Can you work these out from the model? Positions are in its coordinate system, mm. A direction names the side the tool comes from. Coordinates: 2 decimals unless noted, no trailing zeros. Order: outer loops, then holes, each group sorted by start corner. A loop starts at its lowest first (then second) coordinate and runs counter-clockwise, first axis right, second up. Notation, with made-up numbers: (-20, 87) -> (-15, 87) arc R21 cw to (-15, 120) -> close; hole circle Ø10 at (-6.5, 23). An arc over 180 degrees is marked (long way). Answer as CSV lines item,"result".
from build123d import *

# Parameters (mm, degrees)
SKETCH1_W           = 300
SKETCH1_H           = 200
BOSS_EXTRUDE1_DEPTH = 6
SKETCH6_R           = 4
CUT_EXTRUDE2_DEPTH  = 361.605047108
FILLET1_R           = 6.35
SKETCH2_R           = 1.5
CUT_EXTRUDE1_DEPTH  = 361.605047108
SKETCH16_R          = 2.65
M5_THROUGH_DEPTH    = 358.420816406
SKETCH9_R           = 1.5
CUT_EXTRUDE3_DEPTH  = 361.605047108
SKETCH10_R          = 1.5
CUT_EXTRUDE5_DEPTH  = 361.605047108
SKETCH17_R          = 1.6
M3_THROUGH_DEPTH    = 268.189599912
FILLET2_R           = 6.35
MOVE_FACE1_BY       = 0.08
MOVE_FACE1_2_BY     = 0.08
MOVE_FACE1_3_BY     = 0.08
MOVE_FACE1_4_BY     = 0.08
MOVE_FACE1_5_BY     = 0.08
MOVE_FACE1_6_BY     = 0.08
MOVE_FACE1_7_BY     = 0.08
MOVE_FACE1_8_BY     = 0.08
MOVE_FACE1_9_BY     = 0.08
MOVE_FACE1_10_BY    = 0.08
MOVE_FACE1_11_BY    = 0.08
MOVE_FACE1_12_BY    = 0.08
MOVE_FACE1_13_BY    = 0.08
MOVE_FACE1_14_BY    = 0.08
MOVE_FACE1_15_BY    = 0.08
MOVE_FACE1_16_BY    = 0.08
MOVE_FACE1_17_BY    = 0.08
MOVE_FACE1_18_BY    = 0.08
MOVE_FACE1_19_BY    = 0.08
MOVE_FACE1_20_BY    = 0.08
MOVE_FACE1_21_BY    = 0.08
MOVE_FACE1_22_BY    = 0.08
MOVE_FACE1_23_BY    = 0.08
MOVE_FACE1_24_BY    = 0.08
MOVE_FACE1_25_BY    = 0.08
MOVE_FACE1_26_BY    = 0.08


with BuildPart() as part:
    # Sketch1 → Boss-Extrude1 (new body)
    with BuildSketch(Plane(origin=(0, 0, 0), x_dir=(1, 0, 0), z_dir=(0, 1, 0))):
        with Locations((150, 100)):
            Rectangle(SKETCH1_W, SKETCH1_H)
    extrude(amount=BOSS_EXTRUDE1_DEPTH)

    # Sketch6 → Cut-Extrude2 (cut, through all)
    with BuildSketch(Plane(origin=(0, 6, 0), x_dir=(1, 0, 0), z_dir=(0, 1, 0))):
        with Locations(Location((150, 118.651, 0), (0, 0, 270))):
            Circle(SKETCH6_R)
    extrude(amount=-CUT_EXTRUDE2_DEPTH, mode=Mode.SUBTRACT)

    # Fillet1
    fillet1_edges = [part.edges().sort_by_distance(p)[0] for p in [
        (0, 3, -200),
        (300, 3, -200),
        (300, 3, 0),
        (0, 3, 0),
    ]]
    fillet(fillet1_edges, radius=FILLET1_R)

    # Sketch2 → Cut-Extrude1 (cut, through all)
    with BuildSketch(Plane(origin=(0, 6, 0), x_dir=(1, 0, 0), z_dir=(0, 1, 0))):
        with Locations(Location((6.35, 174.6, 0), (0, 0, 270))):
            Circle(SKETCH2_R)
        with Locations(Location((6.35, 49.9999, 0), (0, 0, 270))):
            Circle(SKETCH2_R)
        with Locations(Location((249.2, 75.3999, 0), (0, 0, 270))):
            Circle(SKETCH2_R)
        with Locations(Location((50.8, 75.3999, 0), (0, 0, 270))):
            Circle(SKETCH2_R)
        with Locations(Location((293.65, 49.9999, 0), (0, 0, 270))):
            Circle(SKETCH2_R)
        with Locations(Location((50.8, 24.5999, 0), (0, 0, 270))):
            Circle(SKETCH2_R)
        with Locations(Location((249.2, 24.5999, 0), (0, 0, 270))):
            Circle(SKETCH2_R)
        with Locations(Location((25.4, 193.65, 0), (0, 0, 270))):
            Circle(SKETCH2_R)
        with Locations(Location((274.6, 193.65, 0), (0, 0, 270))):
            Circle(SKETCH2_R)
        with Locations(Location((293.65, 174.6, 0), (0, 0, 270))):
            Circle(SKETCH2_R)
    extrude(amount=-CUT_EXTRUDE1_DEPTH, mode=Mode.SUBTRACT)

    # Sketch16 → M5_through (cut, through all)
    with BuildSketch(Plane(origin=(0, 6, -5.8), x_dir=(1, 0, 0), z_dir=(0, -1, 0))):
        with Locations(Location((118.25, -18.651, 0), (0, 0, 270))):
            Circle(SKETCH16_R)
        with Locations(Location((118.25, -0.55096, 0), (0, 0, 270))):
            Circle(SKETCH16_R)
        with Locations(Location((139.416666667, -0.55096, 0), (0, 0, 270))):
            Circle(SKETCH16_R)
        with Locations(Location((160.583333333, -0.55096, 0), (0, 0, 270))):
            Circle(SKETCH16_R)
        with Locations(Location((181.75, -0.55096, 0), (0, 0, 270))):
            Circle(SKETCH16_R)
        with Locations(Location((181.75, -18.651, 0), (0, 0, 270))):
            Circle(SKETCH16_R)
    extrude(amount=M5_THROUGH_DEPTH, mode=Mode.SUBTRACT)

    # Sketch9 → Cut-Extrude3 (cut, through all)
    with BuildSketch(Plane(origin=(0, 6, 0), x_dir=(-1, 0, 0), z_dir=(0, 1, 0))):
        with Locations(Location((-118.25, -15.40098, 0), (0, 0, 90))):
            Circle(SKETCH9_R)
        with Locations(Location((-150, -6.35096, 0), (0, 0, 90))):
            Circle(SKETCH9_R)
        with Locations(Location((-181.75, -15.40098, 0), (0, 0, 90))):
            Circle(SKETCH9_R)
    extrude(amount=-CUT_EXTRUDE3_DEPTH, mode=Mode.SUBTRACT)

    # Sketch10 → Cut-Extrude5 (cut, through all)
    with BuildSketch(Plane(origin=(0, 6, 0), x_dir=(1, 0, 0), z_dir=(0, 1, 0))):
        with Locations(Location((150, 156.751, 0), (0, 0, 270))):
            Circle(SKETCH10_R)
        with Locations(Location((182.995567884, 137.701, 0), (0, 0, 270))):
            Circle(SKETCH10_R)
        with Locations(Location((182.995567884, 99.601, 0), (0, 0, 270))):
            Circle(SKETCH10_R)
        with Locations(Location((150, 80.551, 0), (0, 0, 270))):
            Circle(SKETCH10_R)
        with Locations(Location((117.004432116, 99.601, 0), (0, 0, 270))):
            Circle(SKETCH10_R)
        with Locations(Location((117.004432116, 137.701, 0), (0, 0, 270))):
            Circle(SKETCH10_R)
        with Locations(Location((105.55, 30.801, 0), (0, 0, 270))):
            Circle(SKETCH10_R)
        with Locations(Location((105.55, 6.35, 0), (0, 0, 270))):
            Circle(SKETCH10_R)
        with Locations(Location((194.45, 6.35, 0), (0, 0, 90))):
            Circle(SKETCH10_R)
        with Locations(Location((194.45, 30.801, 0), (0, 0, 90))):
            Circle(SKETCH10_R)
        with BuildLine():
            Line((124.6, 75.583146559), (124.6, 37.151))
            Line((124.6, 37.151), (92.85, 37.151))
            Line((92.85, 37.151), (92.85, 0))
            Line((92.85, 0), (0, 0))
            Line((0, 0), (0, 200))
            Line((0, 200), (300, 200))
            Line((300, 200), (300, 0))
            Line((300, 0), (207.15, 0))
            Line((207.15, 0), (207.15, 37.151))
            Line((207.15, 37.151), (175.4, 37.151))
            Line((175.4, 37.151), (175.4, 75.583146559))
            ThreePointArc((175.4, 75.583146559), (150, 168.651), (124.6, 75.583146559))
        make_face()
    extrude(amount=-CUT_EXTRUDE5_DEPTH, mode=Mode.SUBTRACT)

    # Sketch17 → M3-through (cut, through all)
    with BuildSketch(Plane(origin=(0, 6, 0), x_dir=(1, 0, 0), z_dir=(0, 1, 0))):
        with Locations(Location((188.1, 118.651, 0), (0, 0, 270))):
            Circle(SKETCH17_R)
        with Locations(Location((169.05, 85.655432116, 0), (0, 0, 270))):
            Circle(SKETCH17_R)
        with Locations(Location((130.95, 85.655432116, 0), (0, 0, 270))):
            Circle(SKETCH17_R)
        with Locations(Location((111.9, 118.651, 0), (0, 0, 270))):
            Circle(SKETCH17_R)
        with Locations(Location((130.95, 151.646567884, 0), (0, 0, 270))):
            Circle(SKETCH17_R)
        with Locations(Location((169.05, 151.646567884, 0), (0, 0, 270))):
            Circle(SKETCH17_R)
    extrude(amount=-M3_THROUGH_DEPTH, mode=Mode.SUBTRACT)

    # Fillet2
    fillet2_edges = [part.edges().sort_by_distance(p)[0] for p in [
        (175.4, 3, -75.583146559),
        (124.6, 3, -75.583146559),
        (124.6, 3, -37.151),
        (92.85, 3, -37.151),
        (92.85, 3, 0),
        (207.15, 3, 0),
        (207.15, 3, -37.151),
        (175.4, 3, -37.151),
    ]]
    fillet(fillet2_edges, radius=FILLET2_R)

    # Move Face1: a curved face moved outward by 0.08
    add(Solid.thicken(part.faces().sort_by_distance((150, 3, -122.651))[0], MOVE_FACE1_BY))

    # Move Face1 2: a curved face moved outward by 0.08
    add(Solid.thicken(part.faces().sort_by_distance((118.25, 3, -21.801))[0], MOVE_FACE1_2_BY))

    # Move Face1 3: a curved face moved outward by 0.08
    add(Solid.thicken(part.faces().sort_by_distance((118.25, 3, -3.70096))[0], MOVE_FACE1_3_BY))

    # Move Face1 4: a curved face moved outward by 0.08
    add(Solid.thicken(part.faces().sort_by_distance((139.416666667, 3, -3.70096))[0], MOVE_FACE1_4_BY))

    # Move Face1 5: a curved face moved outward by 0.08
    add(Solid.thicken(part.faces().sort_by_distance((160.583333333, 3, -3.70096))[0], MOVE_FACE1_5_BY))

    # Move Face1 6: a curved face moved outward by 0.08
    add(Solid.thicken(part.faces().sort_by_distance((181.75, 3, -3.70096))[0], MOVE_FACE1_6_BY))

    # Move Face1 7: a curved face moved outward by 0.08
    add(Solid.thicken(part.faces().sort_by_distance((181.75, 3, -21.801))[0], MOVE_FACE1_7_BY))

    # Move Face1 8: a curved face moved outward by 0.08
    add(Solid.thicken(part.faces().sort_by_distance((118.25, 3, -16.90098))[0], MOVE_FACE1_8_BY))

    # Move Face1 9: a curved face moved outward by 0.08
    add(Solid.thicken(part.faces().sort_by_distance((150, 3, -7.85096))[0], MOVE_FACE1_9_BY))

    # Move Face1 10: a curved face moved outward by 0.08
    add(Solid.thicken(part.faces().sort_by_distance((181.75, 3, -16.90098))[0], MOVE_FACE1_10_BY))

    # Move Face1 11: a curved face moved outward by 0.08
    add(Solid.thicken(part.faces().sort_by_distance((150, 3, -158.251))[0], MOVE_FACE1_11_BY))

    # Move Face1 12: a curved face moved outward by 0.08
    add(Solid.thicken(part.faces().sort_by_distance((182.995567884, 3, -139.201))[0], MOVE_FACE1_12_BY))

    # Move Face1 13: a curved face moved outward by 0.08
    add(Solid.thicken(part.faces().sort_by_distance((182.995567884, 3, -101.101))[0], MOVE_FACE1_13_BY))

    # Move Face1 14: a curved face moved outward by 0.08
    add(Solid.thicken(part.faces().sort_by_distance((150, 3, -82.051))[0], MOVE_FACE1_14_BY))

    # Move Face1 15: a curved face moved outward by 0.08
    add(Solid.thicken(part.faces().sort_by_distance((117.004432116, 3, -101.101))[0], MOVE_FACE1_15_BY))

    # Move Face1 16: a curved face moved outward by 0.08
    add(Solid.thicken(part.faces().sort_by_distance((117.004432116, 3, -139.201))[0], MOVE_FACE1_16_BY))

    # Move Face1 17: a curved face moved outward by 0.08
    add(Solid.thicken(part.faces().sort_by_distance((105.55, 3, -32.301))[0], MOVE_FACE1_17_BY))

    # Move Face1 18: a curved face moved outward by 0.08
    add(Solid.thicken(part.faces().sort_by_distance((105.55, 3, -7.85))[0], MOVE_FACE1_18_BY))

    # Move Face1 19: a curved face moved outward by 0.08
    add(Solid.thicken(part.faces().sort_by_distance((194.45, 3, -4.85))[0], MOVE_FACE1_19_BY))

    # Move Face1 20: a curved face moved outward by 0.08
    add(Solid.thicken(part.faces().sort_by_distance((194.45, 3, -29.301))[0], MOVE_FACE1_20_BY))

    # Move Face1 21: a curved face moved outward by 0.08
    add(Solid.thicken(part.faces().sort_by_distance((188.1, 3, -120.251))[0], MOVE_FACE1_21_BY))

    # Move Face1 22: a curved face moved outward by 0.08
    add(Solid.thicken(part.faces().sort_by_distance((169.05, 3, -87.255432116))[0], MOVE_FACE1_22_BY))

    # Move Face1 23: a curved face moved outward by 0.08
    add(Solid.thicken(part.faces().sort_by_distance((130.95, 3, -87.255432116))[0], MOVE_FACE1_23_BY))

    # Move Face1 24: a curved face moved outward by 0.08
    add(Solid.thicken(part.faces().sort_by_distance((111.9, 3, -120.251))[0], MOVE_FACE1_24_BY))

    # Move Face1 25: a curved face moved outward by 0.08
    add(Solid.thicken(part.faces().sort_by_distance((130.95, 3, -153.246567884))[0], MOVE_FACE1_25_BY))

    # Move Face1 26: a curved face moved outward by 0.08
    add(Solid.thicken(part.faces().sort_by_distance((169.05, 3, -153.246567884))[0], MOVE_FACE1_26_BY))


solid = part.part
Q1. We'd pull the mould along X, two halves only. Please class faces 4 (the flat face through (109, 3, -37.151)), 5 (the cylindrical face through (120.8, 3.04, -6.02)), 6 (the cylindrical face through (184.3, 3.04, -6.02)), 7 (the cylindrical face through (151.78, 3.04, -168.62)): pulls with the +X half, pulls with the -X half, needs draft (parallel to the pull), parting line crosses it, or undercut.
Solution:
face 4,"needs draft"
face 5,"undercut"
face 6,"undercut"
face 7,"parting line crosses it"
Q2. For P1, Ø1.8, axis at x = 130.95, z = -85.66, coming from the +Y side; P2, Ø1, axis at x = 154, y = 4, coming from the -Z side; P3, Ø1.5, axis at x = 157, y = 1.5, coming from the -Z side, each with a flat end and sliding along its axis, tell me the tip position at first contact or that it passes through.
Solution:
P1,"through"
P2,"z = -168.53"
P3,"z = -168.26"
Q3. Which directions (+Z, -Z, +X, -X, +Y, -Y) give clear straight access to the entire face, cutting with the end or side of a thin tool? Please do faces 1 (the cylindrical face through (122.69, 2.96, -38.96)), 2 (the flat face through (191, 3, -37.151)), 3 (the flat face through (151, 0, -86)).
Solution:
face 1,"-X, +Y, -Y"
face 2,"+X, +Y, -Y"
face 3,"+Z, -Z, +X, -X, -Y"
Q4. Imagine slicing it at C-C (z = -34). List the corners of the cut face in (x, y) for me.
Solution:
outline,"(93.71, 0) -> (206.29, 0) -> (206.29, 6) -> (93.71, 6) -> close"
Q5. If I drill on line 1 (Z direction, x = 120.5, y = 4.85); line 2 (X direction, y = 3.65, z = -54.5); line 3 (X direction, y = 2.75, z = -8), over which ranges is the centre line in solid material (lowest first)?
Solution:
line 1,"-159.02 to -78.28, -37.56 to -25.69, -23.21 to -7.59, -5.11 to 0"
line 2,"124.6 to 175.4"
line 3,"92.85 to 116.28, 120.22 to 137.45, 141.39 to 158.61, 162.55 to 179.78, 183.72 to 207.15"
Q6. Imagine slicing it at A-A (y = 1.85). Give the number of separate pieces and of enclosed holes in the cut face, and give its area (3 significant figures).
Solution:
separate pieces,"1"
enclosed holes,"26"
area,"13,500 mm2"
Q7. Imagine slicing it at B-B (z = -141). List the corners of the cut face in (x, y) for me.
Solution:
outline,"(105.27, 0) -> (194.73, 0) -> (194.73, 6) -> (105.27, 6) -> close"
